Check sheet for the modelled part. Datum: model origin and axes. Units: mm. Give positions to 0.01 mm unless a question says otherwise; leave off trailing zeros. Loops run counter-clockwise (first coordinate to the right, second up) from the corner with the lowest first, then second, coordinate; pieces in that order, holes last. Notation, with made-up numbers: M 50,23 L 82,23 A21 ccw 82,30 Z; hole C 87,63 d7. An arc over 180 degrees is marked long. Write each question's results on one line, items separated by ' | '. Start each with the question number.
1. Sectioned sample at A-A on x = 85. Record the cut outline in (y, z), and give its area (3 significant figures).
2. Material ranges on line 1 along X through (y, z) = (4.5, -155); line 2 along Z through (x, y) = (67.5, 5.75); line 3 along X through (y, z) = (5.75, -26), recorded low to high.
3. Draft check along Z on faces 1 (the cylindrical face through (15, 4, -157)), 2 (the flat face through (49, 7, -91)), 3 (the flat face through (49, 3, 0)). Enter one of: pulls with the +Z half, pulls with the -Z half, needs draft (parallel to the pull), parting line crosses it, or undercut.
```python
from build123d import *

# Parameters (mm, degrees)
SKETCH1_W           = 100
SKETCH1_H           = 180
BOSS_EXTRUDE1_DEPTH = 7
SKETCH3_R           = 2
CUT_EXTRUDE1_DEPTH  = 207.031550982
SKETCH4_R           = 1.5
CUT_EXTRUDE2_DEPTH  = 207.031550982


with BuildPart() as part:
    # Sketch1 → Boss-Extrude1 (new body)
    with BuildSketch(Plane(origin=(0, 0, 0), x_dir=(1, 0, 0), z_dir=(0, 1, 0))):
        with Locations((50, 90)):
            Rectangle(SKETCH1_W, SKETCH1_H)
    extrude(amount=BOSS_EXTRUDE1_DEPTH)

    # Sketch3 → Cut-Extrude1 (cut, through all)
    with BuildSketch(Plane(origin=(0, 7, 0), x_dir=(1, 0, 0), z_dir=(0, 1, 0))):
        with Locations(Location((15, 25, 0), (0, 0, 270))):
            Circle(SKETCH3_R)
        with Locations(Location((85, 25, 0), (0, 0, 270))):
            Circle(SKETCH3_R)
        with Locations(Location((15, 155, 0), (0, 0, 270))):
            Circle(SKETCH3_R)
        with Locations(Location((85, 155, 0), (0, 0, 270))):
            Circle(SKETCH3_R)
    extrude(amount=-CUT_EXTRUDE1_DEPTH, mode=Mode.SUBTRACT)

    # Sketch4 → Cut-Extrude2 (cut, through all)
    with BuildSketch(Plane(origin=(0, 7, 0), x_dir=(1, 0, 0), z_dir=(0, 1, 0))):
        with Locations(Location((32.5, 155, 0), (0, 0, 270))):
            Circle(SKETCH4_R)
        with Locations(Location((67.5, 155, 0), (0, 0, 270))):
            Circle(SKETCH4_R)
    extrude(amount=-CUT_EXTRUDE2_DEPTH, mode=Mode.SUBTRACT)


solid = part.part
```
Output values:
1) outline: M 0,-180 L 7,-180 L 7,-157 L 0,-157 Z; M 0,-153 L 7,-153 L 7,-27 L 0,-27 Z; M 0,-23 L 7,-23 L 7,0 L 0,0 Z | area: 1,200 mm2
2) line 1: 0 to 13, 17 to 31, 34 to 66, 69 to 83, 87 to 100 | line 2: -180 to -156.5, -153.5 to 0 | line 3: 0 to 13.27, 16.73 to 83.27, 86.73 to 100
3) face 1: undercut | face 2: needs draft | face 3: pulls with the +Z half
